For this review, use the dimensioned drawing (mm, ordinates from the lowest corner) and the shaded views. Give positions to 0.01 mm unless a question says otherwise; leave off trailing zeros. Write each loop counter-clockwise with the first axis right and the second up, starting at its lowest first coordinate (ties: lowest second). Pieces come first, ordered by that corner, then holes. Notation, with made-up numbers: M -14.5,-30.5 L 17.5,-30.5 A22 cw 17.5,-14.5 Z; hole C 72.25,27.25 d2. An arc over 180 degrees is marked long. Answer in a Markdown table with one row per item.
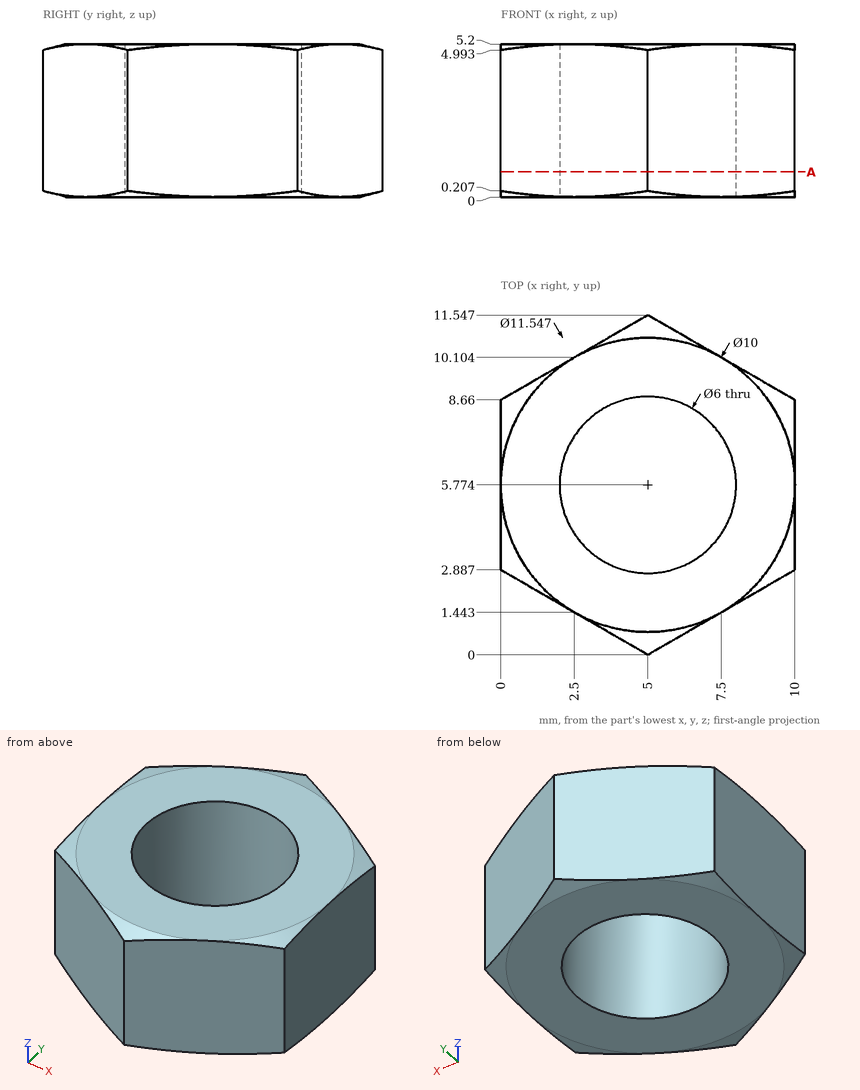
1) To check wall thickness, follow probe 1 along X at (y, z) = (7.75, 2.95) (1 decimal); probe 2 along Y at (x, z) = (5.5, 2.4) (1 decimal); probe 3 along Y at (x, z) = (6, 3.05) (1 decimal). State the ranges of each line that lie inside material, in increasing order. Write a range as [from, to].
Geometry says:
| item | result |
|---|---|
| probe 1 | [0, 2.7], [7.3, 10] |
| probe 2 | [0.3, 2.8], [8.7, 11.3] |
| probe 3 | [0.6, 2.9], [8.6, 11] |
2) Add section A-A (z = 0.85). Write out the cut boundary in (x, y).
Geometry says:
| item | result |
|---|---|
| outline | M 0,2.89 L 5,0 L 10,2.89 L 10,8.66 L 5,11.55 L 0,8.66 Z; hole C 5,5.77 d6 |
3) Insertion check: P1, Ø3.5, axis at x = 5, y = 5.77, coming from the +Z side; P2, Ø2, axis at x = 7.5, z = 2, coming from the -Y side (1 decimal). Each pin has a flat end and moves straight along its axis. Give the tip position at first contact, or say it passes through.
Geometry says:
| item | result |
|---|---|
| P1 | through |
| P2 | y = 0.9 |
